Design review of the part built by this model. Coordinates are the model's own, in mm. A direction names the side the tool comes from. Coordinates: 2 decimals unless noted, no trailing zeros. Order: outer loops, then holes, each group sorted by start corner. A loop starts at its lowest first (then second) coordinate and runs counter-clockwise, first axis right, second up. Notation, with made-up numbers: M 32,68 L 52,68 A23 ccw 52,90 Z; hole C -27,-25.5 d5. An arc over 180 degrees is marked long. Answer in a Markdown table with one row per item.
from build123d import *

# Parameters (mm, degrees)
F0_W     = 1230
F0_H     = 700
F1_DEPTH = 40
F3_T     = -10
F4_R     = 30


with BuildPart() as f1:
    # F0 (on Front) → F1 (new body)
    with BuildSketch(Plane.XZ):
        with Locations((7.912883, 14.9518)):
            Rectangle(F0_W, F0_H)
    extrude(amount=F1_DEPTH)

    # F3
    f3_openings = [f1.faces().sort_by_distance(p)[0] for p in [
        (7.912883, -40, 14.9518),
    ]]
    offset(amount=F3_T, openings=f3_openings)

    # F4
    f4_edges = [f1.edges().sort_by_distance(p)[0] for p in [
        (7.912883, 0, -335.0482),
        (7.912883, 0, 364.9518),
        (-607.087117, 0, 14.9518),
        (622.912883, 0, 14.9518),
    ]]
    fillet(f4_edges, radius=F4_R)


solid = f1.part
(1) Draft analysis for pull direction Z (two halves, no side actions). For faces 1 (the flat face through (-597.087, -25, 10)), 2 (the cylindrical face through (16.523, -9.021, 356.397)), 3 (the cylindrical face through (-598.53, -9.02, 19.85)), state which applies: pulls with the +Z half, pulls with the -Z half, needs draft (parallel to the pull), parting line crosses it, or undercut.
Return value:
| item | result |
|---|---|
| face 1 | undercut |
| face 2 | pulls with the +Z half |
| face 3 | needs draft |
(2) Add section B-B, the plane y = -16.5. Give the boundary of the cut face in (x, z), and give its area (3 significant figures).
Return value:
| item | result |
|---|---|
| outline | M -603.88,-331.84 L 619.7,-331.84 L 619.7,361.74 L -603.88,361.74 Z; hole M -597.09,-325.05 L 612.91,-325.05 L 612.91,354.95 L -597.09,354.95 Z |
| area | 25,900 mm2 |
(3) Add section C-C, the plane z = -199. Give the boundary of the cut face in (x, y).
Return value:
| item | result |
|---|---|
| outline | M -607.09,-40 L -597.09,-40 L -597.09,-10 L 612.91,-10 L 612.91,-40 L 622.91,-40 L 622.91,-30 A30 ccw 592.91,0 L -577.09,0 A30 ccw -607.09,-30 Z |
(4) Add section A-A, the plane x = -30. Give the boundary of the cut face in (y, z).
Return value:
| item | result |
|---|---|
| outline | M -40,-335.05 L -30,-335.05 A30 ccw 0,-305.05 L 0,334.95 A30 ccw -30,364.95 L -40,364.95 L -40,354.95 L -10,354.95 L -10,-325.05 L -40,-325.05 Z |
(5) For line 1 along Z through (x, y) = (-412.5, -28.5); line 2 along X through (y, z) = (-28.5, -73); line 3 along X through (y, z) = (-37.5, 230), list the stretches that pass through material, from the lowest coordinate up. Write a range as from..to.
Return value:
| item | result |
|---|---|
| line 1 | z = -335.01..-325.05, 354.95..364.91 |
| line 2 | x = -607.05..-597.09, 612.91..622.88 |
| line 3 | x = -607.09..-597.09, 612.91..622.91 |
(6) For faces 4 (the flat face through (-1, -25, -325.048)), 5 (the flat face through (0, 0, 19)), list the 3-axis set-ups (+Z, -Z, +X, -X, +Y, -Y) from which the entire face can be reached by the end or side of a thin tool; tool diameter is ignored.
Return value:
| item | result |
|---|---|
| face 4 | -Y |
| face 5 | +Z, -Z, +X, -X, +Y |
(7) Insertion check: pin 1 Ø6 at (y, z) = (-18, 241.5) entering from +X; pin 2 Ø24 at (x, y) = (298, -25) entering from -Z; pin 3 Ø9 at (y, z) = (-21.5, -3.5) entering from +X (3 decimals); pin 4 Ø5 at (x, y) = (409, -23) entering from -Z. Each pin has a flat end and moves straight along its axis. Give the tip position at first contact, or say it passes through.
Return value:
| item | result |
|---|---|
| pin 1 | stops at x = 621.53 |
| pin 2 | stops at z = -335.05 |
| pin 3 | stops at x = 622.645 |
| pin 4 | stops at z = -334.71 |
